The listing builds one solid part. Answer for the finished solid, in the listing's coordinates (mm). Give positions to 0.01 mm unless a question says otherwise; leave off trailing zeros. Order: outer loops, then holes, each group sorted by start corner. A loop starts at its lowest first (then second) coordinate and runs counter-clockwise, first axis right, second up. Notation, with made-up numbers: (-21, -18) - (17, -18) arc R36 cw to (17, 18) - close; hole circle Ø9 at (79, 39). An arc over 180 degrees is marked (long way). Write each question's results on one line, items separated by ' | '. Start each with the question number.
1. Find the intervals of material crossed by L1, parallel to Y at x = 66.5, z = 3.5; L2, parallel to X at y = 12, z = 5.25, in increasing order.
2. Flat-ended cylindrical pins translate along their axes: pin 1 (10 mm diameter, centred on x = 39.5, y = 31.5, fed in from -Z); pin 2 (1.9 mm diameter, centred on y = 18.5, z = 2, fed in from -X). Find the tip coordinate at first contact, or state that the pin passes through.
3. Section B-B (y = 28) is taken. Give the vertices of the cut face in (x, z).
4. Section A-A (z = 1.5) is taken. Give the vertices of the cut face in (x, y), and give its area (3 significant figures).
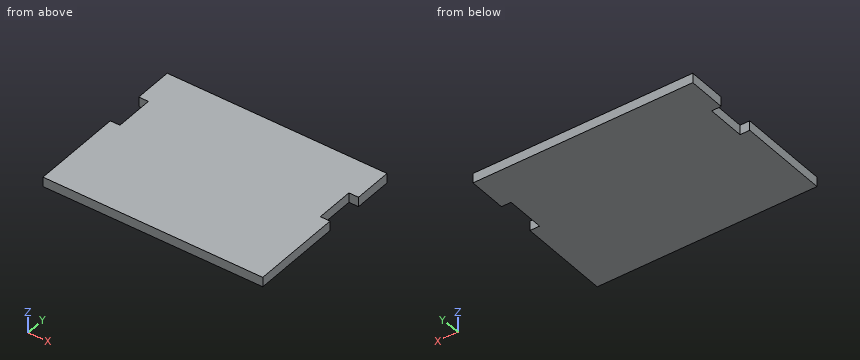
from build123d import *

# Parameters (mm, degrees)
SKETCH1_W           = 144.78
SKETCH1_H           = 114.3
BOSS_EXTRUDE1_DEPTH = 6.35
CAVITY1_START       = -72.39
CAVITY1_OUTLINE_W   = 25.4
CAVITY1_OUTLINE_H   = 6.35
CAVITY1_DEPTH       = 6.35
CAVITY1_START_2     = 66.04
CAVITY1_2_OUTLINE_W = 25.4
CAVITY1_2_OUTLINE_H = 6.35
CAVITY1_2_DEPTH     = 6.35
SKETCH4_W           = 144.78
SKETCH4_H           = 3.477037696
CUT_EXTRUDE2_DEPTH  = 93.448672787


# Read off the part's stored shape, not the designer's step: Cavity1
with BuildPart() as part:
    # Sketch1 → Boss-Extrude1 (new body)
    with BuildSketch(Plane.XY):
        Rectangle(SKETCH1_W, SKETCH1_H)
    extrude(amount=BOSS_EXTRUDE1_DEPTH)

    # Cavity1 outline → Cavity1 (cut)
    with BuildSketch(Plane.YZ.offset(CAVITY1_START)):
        with Locations((19.05, 3.175)):
            Rectangle(CAVITY1_OUTLINE_W, CAVITY1_OUTLINE_H)
    extrude(amount=CAVITY1_DEPTH, mode=Mode.SUBTRACT)

    # Cavity1 2 outline → Cavity1 2 (cut)
    with BuildSketch(Plane.YZ.offset(CAVITY1_START_2)):
        with Locations((19.05, 3.175)):
            Rectangle(CAVITY1_2_OUTLINE_W, CAVITY1_2_OUTLINE_H)
    extrude(amount=CAVITY1_2_DEPTH, mode=Mode.SUBTRACT)

    # Sketch4 → Cut-Extrude2 (cut, through all)
    with BuildSketch(Plane.XY.offset(6.35)):
        with Locations((0, -55.411481152)):
            Rectangle(SKETCH4_W, SKETCH4_H)
    extrude(amount=-CUT_EXTRUDE2_DEPTH, mode=Mode.SUBTRACT)


solid = part.part
Reported:
1) L1: -53.67 to 6.35, 31.75 to 57.15 | L2: -66.04 to 66.04
2) pin 1: z = 0 | pin 2: x = -66.04
3) outline: (-66.04, 0) - (66.04, 0) - (66.04, 6.35) - (-66.04, 6.35) - close
4) outline: (-72.39, -53.67) - (72.39, -53.67) - (72.39, 6.35) - (66.04, 6.35) - (66.04, 31.75) - (72.39, 31.75) - (72.39, 57.15) - (-72.39, 57.15) - (-72.39, 31.75) - (-66.04, 31.75) - (-66.04, 6.35) - (-72.39, 6.35) - close | area: 15,700 mm²
